```python
from build123d import *

# Parameters (mm, degrees)
EXTRUDE_1_DEPTH     = 3
SKETCH_4_W          = 3
SKETCH_4_H          = 3.704951288
EXTRUDE_3_DEPTH     = 1
CUT_EXTRUDE_2_REACH = 25.05
SKETCH_6_R          = 0.5
CUT_EXTRUDE_3_DEPTH = 3


with BuildPart() as part:
    # Sketch 1 → Extrude 1 (new body)
    with BuildSketch(Plane.XY):
        with BuildLine():
            ThreePointArc((-4.975392322, 2.84990406), (-4.993840493, 2.675384142), (-5, 2.5))
            Line((-5, 2.5), (-5, -1.5))
            Line((-5, -1.5), (-5, -2.5))
            ThreePointArc((-5, -2.5), (-4.993840493, -2.675384142), (-4.975392322, -2.84990406))
            ThreePointArc((-4.975392322, -2.84990406), (-3.464823228, -3.464823228), (-2.84990406, -4.975392322))
            ThreePointArc((-2.84990406, -4.975392322), (-2.675384142, -4.993840493), (-2.5, -5))
            Line((-2.5, -5), (-1.5, -5))
            Line((-1.5, -5), (2.5, -5))
            ThreePointArc((2.5, -5), (2.675384142, -4.993840493), (2.84990406, -4.975392322))
            ThreePointArc((2.84990406, -4.975392322), (3.464823228, -3.464823228), (4.975392322, -2.84990406))
            ThreePointArc((4.975392322, -2.84990406), (4.993840493, -2.675384142), (5, -2.5))
            Line((5, -2.5), (5, 1.5))
            Line((5, 1.5), (5, 2.5))
            ThreePointArc((5, 2.5), (4.993840493, 2.675384142), (4.975392322, 2.84990406))
            ThreePointArc((4.975392322, 2.84990406), (3.464823228, 3.464823228), (2.84990406, 4.975392322))
            ThreePointArc((2.84990406, 4.975392322), (2.675384142, 4.993840493), (2.5, 5))
            Line((2.5, 5), (1.5, 5))
            Line((1.5, 5), (-2.5, 5))
            ThreePointArc((-2.5, 5), (-2.675384142, 4.993840493), (-2.84990406, 4.975392322))
            ThreePointArc((-2.84990406, 4.975392322), (-3.464823228, 3.464823228), (-4.975392322, 2.84990406))
        make_face()
        with BuildLine():
            ThreePointArc((-3.5, 2.5), (-3.207106781, 3.207106781), (-2.5, 3.5))
            Line((-2.5, 3.5), (2.5, 3.5))
            ThreePointArc((2.5, 3.5), (3.207106781, 3.207106781), (3.5, 2.5))
            Line((3.5, 2.5), (3.5, -2.5))
            ThreePointArc((3.5, -2.5), (3.207106781, -3.207106781), (2.5, -3.5))
            Line((2.5, -3.5), (-2.5, -3.5))
            ThreePointArc((-2.5, -3.5), (-3.207106781, -3.207106781), (-3.5, -2.5))
            Line((-3.5, -2.5), (-3.5, 2.5))
        make_face(mode=Mode.SUBTRACT)
        with BuildLine():
            Line((-5, -2.5), (-5, -1.5))
            ThreePointArc((-5, -1.5), (-5.161755993, -2.313202294), (-5.62239809, -3.00260191))
            Line((-5.62239809, -3.00260191), (-8.450825215, -5.831029035))
            Line((-8.450825215, -5.831029035), (-5.831029035, -8.450825215))
            Line((-5.831029035, -8.450825215), (-3.00260191, -5.62239809))
            ThreePointArc((-3.00260191, -5.62239809), (-2.313202294, -5.161755993), (-1.5, -5))
            Line((-1.5, -5), (-2.5, -5))
            ThreePointArc((-2.5, -5), (-2.675384142, -4.993840493), (-2.84990406, -4.975392322))
            ThreePointArc((-2.84990406, -4.975392322), (-4.267766953, -4.267766953), (-4.975392322, -2.84990406))
            ThreePointArc((-4.975392322, -2.84990406), (-4.993840493, -2.675384142), (-5, -2.5))
        make_face()
        with BuildLine():
            ThreePointArc((3.00260191, 5.62239809), (2.313202294, 5.161755993), (1.5, 5))
            Line((1.5, 5), (2.5, 5))
            ThreePointArc((2.5, 5), (2.675384142, 4.993840493), (2.84990406, 4.975392322))
            ThreePointArc((2.84990406, 4.975392322), (4.267766953, 4.267766953), (4.975392322, 2.84990406))
            ThreePointArc((4.975392322, 2.84990406), (4.993840493, 2.675384142), (5, 2.5))
            Line((5, 2.5), (5, 1.5))
            ThreePointArc((5, 1.5), (5.161755993, 2.313202294), (5.62239809, 3.00260191))
            Line((5.62239809, 3.00260191), (8.450825215, 5.831029035))
            Line((8.450825215, 5.831029035), (5.831029035, 8.450825215))
            Line((5.831029035, 8.450825215), (3.00260191, 5.62239809))
        make_face()
    extrude(amount=EXTRUDE_1_DEPTH)

    # Sketch 4 → Extrude 3 (add)
    with BuildSketch(Plane(origin=(-7.140927125, -7.140927125, 0), x_dir=(0, 0, 1), z_dir=(-0.707106781, -0.707106781, 0))):
        with Locations((1.5, 0)):
            Rectangle(SKETCH_4_W, SKETCH_4_H)
    extrude(amount=EXTRUDE_3_DEPTH)

    # Sketch 6 → Cut-Extrude 2 (cut, up to next)
    with BuildSketch(Plane(origin=(7.140927125, 7.140927125, 0), x_dir=(0, 0, -1), z_dir=(0.707106781, 0.707106781, 0)), mode=Mode.PRIVATE) as cut_extrude_2_sk1:
        with Locations((-1.5, 0)):
            Circle(SKETCH_6_R)
    cut_extrude_2_tool1 = extrude(cut_extrude_2_sk1.sketch, amount=-CUT_EXTRUDE_2_REACH, mode=Mode.PRIVATE) & part.part
    add(cut_extrude_2_tool1.solids().sort_by_distance((7.140927, 7.140927, 1.5))[0], mode=Mode.SUBTRACT)

    # Sketch 7 → Cut-Extrude 3 (cut)
    with BuildSketch(Plane(origin=(0, 0, 0), x_dir=(-1, 0, 0), z_dir=(0, 0, -1))):
        with BuildLine():
            ThreePointArc((7.939042101, -7.118737583), (7.844102323, -7.544021013), (7.57731011, -7.888551813))
            Line((7.57731011, -7.888551813), (6.315197686, -8.934993866))
            Line((6.315197686, -8.934993866), (6.538135816, -9.157931996))
            Line((6.538135816, -9.157931996), (9.157931996, -6.538135816))
            Line((9.157931996, -6.538135816), (6.179905917, -3.560109737))
            Line((6.179905917, -3.560109737), (5.226626879, -4.513388774))
            Line((5.226626879, -4.513388774), (6.357997729, -5.644759624))
            ThreePointArc((6.357997729, -5.644759624), (6.40623087, -5.695293259), (6.452058903, -5.748017783))
            Line((6.452058903, -5.748017783), (6.771192907, -6.132924899))
            ThreePointArc((6.771192907, -6.132924899), (7.584081172, -6.354587992), (7.939042101, -7.118737583))
        make_face()
        with BuildLine():
            Line((6.315197686, -8.934993866), (7.57731011, -7.888551813))
            ThreePointArc((7.57731011, -7.888551813), (6.913068809, -8.11840022), (6.26165953, -7.854368504))
            ThreePointArc((6.26165953, -7.854368504), (5.933311195, -8.06392542), (5.56207655, -8.18187273))
            Line((5.56207655, -8.18187273), (6.315197686, -8.934993866))
        make_face()
        with BuildLine():
            ThreePointArc((5.56207655, -8.18187273), (5.933311195, -8.06392542), (6.26165953, -7.854368504))
            ThreePointArc((6.26165953, -7.854368504), (5.96671976, -7.352381038), (6.001378676, -6.771192907))
            Line((6.001378676, -6.771192907), (5.682244672, -6.386285792))
            ThreePointArc((5.682244672, -6.386285792), (5.853125459, -6.685300378), (5.912430442, -7.0245538))
            ThreePointArc((5.912430442, -7.0245538), (5.750922734, -7.569467258), (5.318569088, -7.938365268))
            Line((5.318569088, -7.938365268), (5.56207655, -8.18187273))
        make_face()
        with BuildLine():
            ThreePointArc((4.142616197, -7.662821791), (4.684294436, -7.998183074), (5.318569088, -7.938365268))
            Line((5.318569088, -7.938365268), (3.998618973, -6.618415153))
            ThreePointArc((3.998618973, -6.618415153), (3.921801757, -7.161136406), (4.142616197, -7.662821791))
        make_face()
        with BuildLine():
            Line((3.998618973, -6.618415153), (5.318569088, -7.938365268))
            ThreePointArc((5.318569088, -7.938365268), (5.750922734, -7.569467258), (5.912430442, -7.0245538))
            ThreePointArc((5.912430442, -7.0245538), (5.853125459, -6.685300378), (5.682244672, -6.386285792))
            ThreePointArc((5.682244672, -6.386285792), (5.65169265, -6.351136109), (5.619537223, -6.317447019))
            ThreePointArc((5.619537223, -6.317447019), (4.729873159, -6.041358581), (3.998618973, -6.618415153))
        make_face()
        with BuildLine():
            Line((3.820884623, -6.440680803), (3.998618973, -6.618415153))
            ThreePointArc((3.998618973, -6.618415153), (4.729873159, -6.041358581), (5.619537223, -6.317447019))
            Line((5.619537223, -6.317447019), (4.652967038, -5.350876834))
            ThreePointArc((4.652967038, -5.350876834), (4.105116436, -5.795140279), (3.820884623, -6.440680803))
        make_face()
        with BuildLine():
            Line((3.560109737, -6.179905917), (3.820884623, -6.440680803))
            ThreePointArc((3.820884623, -6.440680803), (4.105116436, -5.795140279), (4.652967038, -5.350876834))
            Line((4.652967038, -5.350876834), (4.521052929, -5.218962725))
            Line((4.521052929, -5.218962725), (3.560109737, -6.179905917))
        make_face()
    extrude(amount=-CUT_EXTRUDE_3_DEPTH, mode=Mode.SUBTRACT)


solid = part.part
```
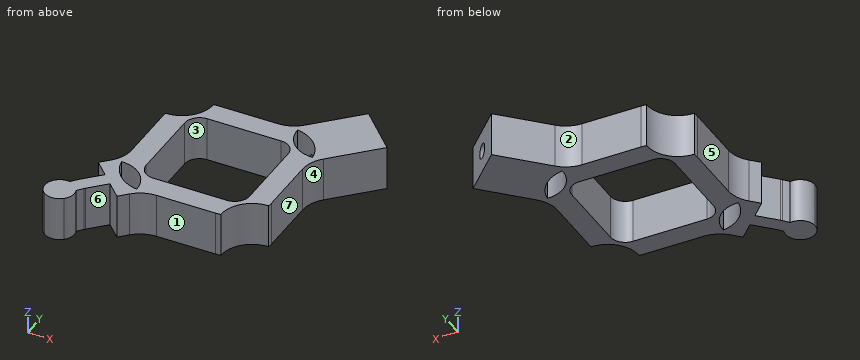
Check sheet for the modelled part. Datum: model origin and axes. Units: mm. Face numbers are marked on the shaded views. A direction names the side the tool comes from. Coordinates: 2 decimals unless noted, no trailing zeros. Loops run counter-clockwise (first coordinate to the right, second up) from the corner with the lowest first, then second, coordinate; pieces in that order, holes last.
1) Gauge pin test, flat ends, axial feed: pin 1 (0.9 mm diameter, centred on y = 1, z = 2, fed in from +X); pin 2 (1.5 mm diameter, centred on x = 1, y = 6.5, fed in from +Z); pin 3 (1.5 mm diameter, centred on y = 0.5, z = 1.5, fed in from -X); pin 4 (1.5 mm diameter, centred on x = 4, z = 1.5, fed in from +Y). Record the tip position at first contact, or that the pin passes through.
2) Access from +Z, -Z, +X, -X, +Y, -Y to the whole of each face (thin tool, end or side, straight path). Record for the marked faces 5, 6 and 7.
3) Material ranges on probe 1 along X at (y, z) = (-1.5, 2.5); probe 2 along X at (y, z) = (-4.75, 2.65), recorded low to high.
4) Release check for a two-part mould opening along X. For the marked faces 1, 2, 3 and 4 record: released by +X, released by -X, zero draft, split by the parting line, or undercut.
5) Sectioned sample at C-C (z = 2.55). Count the separate pieces of the cut face and the enclosed holes in it, and give its area (3 significant figures).
6) Sectioned sample at A-A (y = -1). Record the boundary of the cut face in (x, z).
Check sheet entries:
1. pin 1: stops at x = 5
1. pin 2: passes through
1. pin 3: stops at x = -5
1. pin 4: stops at y = 7.37
2. face 5: +Z, -Z, -X, +Y
2. face 6: +Z, -Z, -Y
2. face 7: +Z, -Z, +X, -Y
3. probe 1: x = -5 to -3.5, 3.5 to 5
3. probe 2: x = -5.46 to -3.59, -2.86 to 2.86
4. face 1: zero draft
4. face 2: released by -X
4. face 3: undercut
4. face 4: released by +X
5. separate pieces: 1
5. enclosed holes: 3
5. area: 62.8 mm2
6. outline: (-5, 0) - (-3.5, 0) - (-3.5, 3) - (-5, 3) - close; (3.5, 0) - (5, 0) - (5, 3) - (3.5, 3) - close
